The figure shows three views and two pictorial views of one solid part (mm, origin at its lowest corner). Answer the questions. A direction names the side the tool comes from. Coordinates: 2 decimals unless noted, no trailing zeros. Order: outer loops, then holes, each group sorted by start corner. A loop starts at its lowest first (then second) coordinate and runs counter-clockwise, first axis right, second up. Notation, with made-up numbers: M 75.25,82 L 111.25,82 A21 cw 111.25,90 Z; hole C 37.5,18.5 d10. An arc over 180 degrees is marked long. Answer in a Markdown table with one row per item. Add a question column.
Item 1: The part is cut by section C-C (y = 2.5). Write down the section's boundary in (x, z).
Item 2: The part is cut by section A-A (x = 13.5). Write down the section's boundary in (y, z).
Item 3: The part is cut by section D-D (x = 5.75). Write down the section's boundary in (y, z).
Item 4: Which of the six approach directions +Z, -Z, +X, -X, +Y, -Y give full straight-line access (tool end or side, diameter ignored) to the marked faces 4 and 5?
Item 5: The part is cut by section B-B (z = 13.5). Write down the section's boundary in (x, y), then the cut area to 3 significant figures.
Item 6: A flat-ended cylindrical pin translates along its axis: pin 1 Ø1.4 at (x, z) = (7, 14) entering from +Y. Find the tip coordinate at first contact, or state that the pin passes through.
Item 7: The mould has two halves that part along Z. Classify the marked faces 1, 2 and 3: released by +Z, released by -Z, zero draft, split by the parting line, or undercut.
Item 8: Consider line 1 (X direction, y = 3.45, z = 13.5); line 2 (X direction, y = 1.55, z = 13); line 3 (Z direction, x = 6.75, y = 2.9). Determine where each line is inside the solid, lowest interval first. Write a range as from..to.
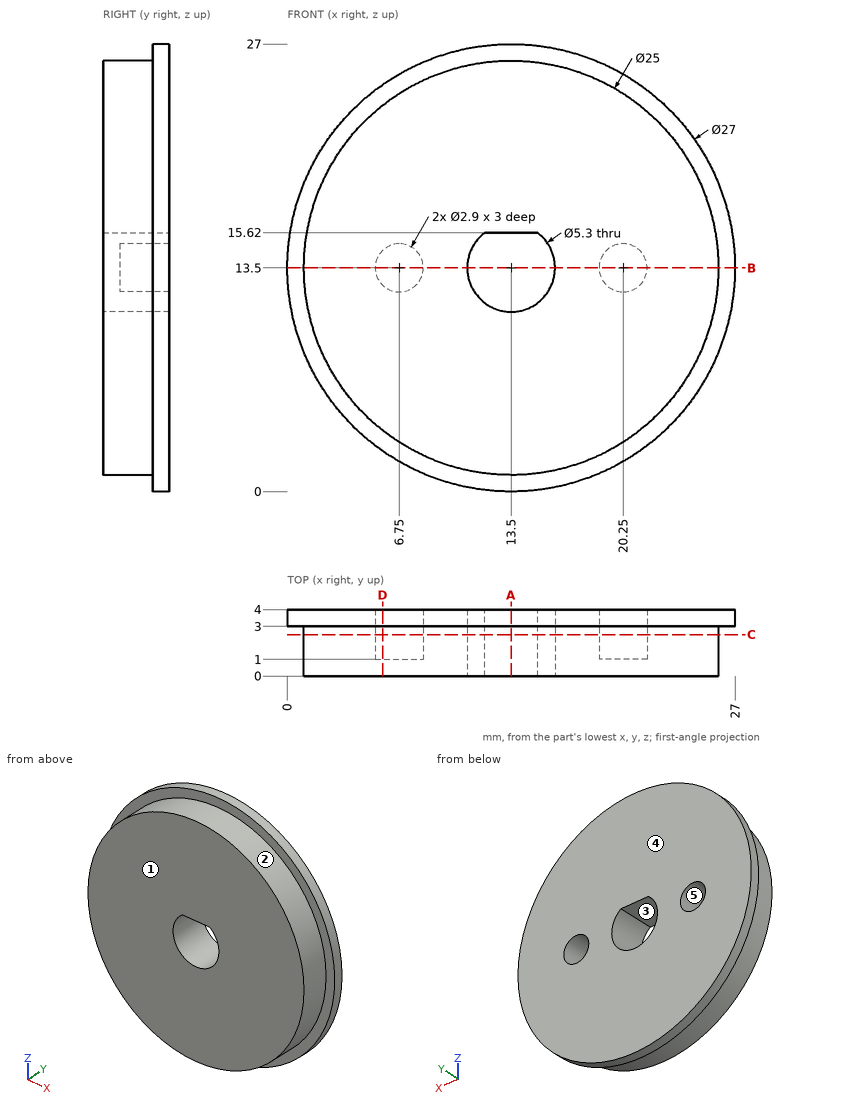
Reply:
| question | item | result |
|---|---|---|
| 1 | outline | C 13.5,13.5 d25; hole C 6.75,13.5 d2.9; hole M 11.91,15.62 A2.65 ccw long 15.09,15.62 Z; hole C 20.25,13.5 d2.9 |
| 2 | outline | M 0,1 L 3,1 L 3,0 L 4,0 L 4,10.85 L 0,10.85 Z; M 0,15.62 L 4,15.62 L 4,27 L 3,27 L 3,26 L 0,26 Z |
| 3 | outline | M 0,3.69 L 3,3.69 L 3,2.45 L 4,2.45 L 4,12.45 L 1,12.45 L 1,14.55 L 4,14.55 L 4,24.55 L 3,24.55 L 3,23.31 L 0,23.31 Z |
| 4 | face 4 | +Z, -Z, +X, -X, +Y |
| 4 | face 5 | +Y |
| 5 | outline | M 0,3 L 1,3 L 1,0 L 10.85,0 L 10.85,4 L 8.2,4 L 8.2,1 L 5.3,1 L 5.3,4 L 0,4 Z; M 16.15,0 L 26,0 L 26,3 L 27,3 L 27,4 L 21.7,4 L 21.7,1 L 18.8,1 L 18.8,4 L 16.15,4 Z |
| 5 | area | 63.4 mm2 |
| 6 | pin 1 | stops at y = 1 |
| 7 | face 1 | zero draft |
| 7 | face 2 | split by the parting line |
| 7 | face 3 | undercut |
| 8 | line 1 | x = 0..5.3, 8.2..10.85, 16.15..18.8, 21.7..27 |
| 8 | line 2 | x = 1.01..5.39, 8.11..10.9, 16.1..18.89, 21.61..25.99 |
| 8 | line 3 | z = 2.98..12.05, 14.95..24.02 |
